from build123d import *

# Parameters (mm, degrees)
BOSS_EXTRUDE1_DEPTH            = 3
SKETCH2_W                      = 2.725
SKETCH2_H                      = 93.5
REVOLVE1_ANGLE                 = 180
SKETCH2_3_W                    = 1.7
SKETCH2_3_H                    = 93.5
M4_CLEARANCE_HOLE1_D           = 4.5
M4_CLEARANCE_HOLE1_CSINK_D     = 4.55
M4_CLEARANCE_HOLE1_CSINK_ANGLE = 90
FILLET1_R                      = 4
FILLET2_R                      = 2.5
CUT_EXTRUDE2_DEPTH             = 5


with BuildPart() as part:
    # Sketch1 → Boss-Extrude1 (new body)
    with BuildSketch(Plane.XY):
        Polygon((-22, 0), (22, 0), (22, -10), (40, -10), (40, -39.5), (24.672961021, -39.5), (12, -71.5), (-12, -71.5), (-24.672961021, -39.5), (-40, -39.5), (-40, -10), (-22, -10), align=None)
    extrude(amount=BOSS_EXTRUDE1_DEPTH)

    # Sketch2 → Revolve1 (revolve)
    with BuildSketch(Plane.XY):
        with Locations((-3.0625, -118.25)):
            Rectangle(SKETCH2_W, SKETCH2_H)
        Polygon((-4.425, -40), (-4.425, -71.5), (-1.7, -71.5), (-1.7, -34), (-4.425, -34), (-4.425, 0), (-10, 0), (-10, -30), align=None)
    revolve(axis=Axis((0, 0, 0), (0, 1, 0)), revolution_arc=REVOLVE1_ANGLE)

    # Sketch2<3> → Cut-Revolve1 (revolve, cut)
    with BuildSketch(Plane.XY):
        with Locations((-0.85, -118.25)):
            Rectangle(SKETCH2_3_W, SKETCH2_3_H)
        Polygon((-1.7, -34), (-1.7, -71.5), (0, -71.5), (0, 0), (-4.425, 0), (-4.425, -34), align=None)
    revolve(axis=Axis((0, 0, 0), (0, -1, 0)), mode=Mode.SUBTRACT)

    # M4 Clearance Hole1 (through all)
    with Locations(Plane.XY.offset(3)):
        with Locations((-35.5, -14.5), (-9, -66.5), (9, -66.5), (35.5, -14.5)):
            CounterSinkHole(M4_CLEARANCE_HOLE1_D / 2, M4_CLEARANCE_HOLE1_CSINK_D / 2, counter_sink_angle=M4_CLEARANCE_HOLE1_CSINK_ANGLE)

    # Fillet1
    # the kernel refuses this fillet: 4 mm, written as the material it adds along each edge
    with BuildSketch(Plane(origin=(0, -34, 0), x_dir=(1, 0, 0), z_dir=(0, 0, -1))) as fillet1_piece_1:
        with BuildLine():
            CenterArc((0.425, -3.791355299), FILLET1_R, 0, 71.412652979)
            Line((1.7, 0), (1.7255, 0.075827106))
            ThreePointArc((1.7255, 0.075827106), (3.0625, 0.08), (4.425, 0.08))
            Line((4.425, 0.08), (4.505, 0))
            Line((4.505, 0), (4.505, -3.791355299))
            Line((4.505, -3.791355299), (4.425, -3.791355299))
        make_face()
    revolve(axis=Axis((0, -34, 0), (0, -1, 0)), revolution_arc=180)

    # Fillet2
    fillet2_edges = [part.edges().sort_by_distance(p)[0] for p in [
        (-22, 0, 1.5),
        (22, 0, 1.5),
        (22, -10, 1.5),
        (40, -10, 1.5),
        (40, -39.5, 1.5),
        (24.672961021, -39.5, 1.5),
        (12, -71.5, 1.5),
        (-12, -71.5, 1.5),
        (-24.672961021, -39.5, 1.5),
        (-40, -39.5, 1.5),
        (-40, -10, 1.5),
        (-22, -10, 1.5),
        (4.121541499, -71.5, 1.610441142),
        (-4.121541499, -71.5, 1.610441142),
    ]]
    fillet(fillet2_edges, radius=FILLET2_R)

    # Sketch9 → Cut-Extrude2 (cut, symmetric)
    with BuildSketch(Plane(origin=(0, 0, 0), x_dir=(0, 0, -1), z_dir=(1, 0, 0))):
        Polygon((-4.425, -162), (4.425, -165), (-4.425, -165), align=None)
    extrude(amount=CUT_EXTRUDE2_DEPTH, both=True, mode=Mode.SUBTRACT)


solid = part.part
Build history of the part. All positions in model axes, mm. A direction names the side the tool comes from. Coordinates: 2 decimals unless noted, no trailing zeros. Order: outer loops, then holes, each group sorted by start corner. A loop starts at its lowest first (then second) coordinate and runs counter-clockwise, first axis right, second up. Notation, with made-up numbers: (-10.75, 9.25) -> (10.25, 9.25) arc R23 cw to (10.25, 28.25) -> close; hole circle Ø11 at (60, 75.5). An arc over 180 degrees is marked (long way). One line per item, written item: value.
(1) Tool access for faces 5 (the cylindrical face through (0.097, -15.316, 4.424)), 6 (the flat face through (-22, -5, 1)), 7 (the flat face through (22, -5, 1)): list every direction of +Z, -Z, +X, -X, +Y, -Y with a clear straight run to the whole face (end or side of a thin tool).
Checked values:
face 5: -Z, +Y
face 6: +Z, -Z, -X, +Y
face 7: +Z, -Z, +X, +Y
(2) Mould opens along Y. For faces 1 (the cylindrical face through (33.42, -15.36, 1.47)), 2 (the flat face through (-9, -71.5, 1)), 3 (the flat face through (40, -25, 1)), 4 (the cylindrical face through (-37.58, -15.36, 1.47)) say: pulls with the +Y half, pulls with the -Y half, needs draft (parallel to the pull), parting line crosses it, or undercut.
Checked values:
face 1: undercut
face 2: pulls with the -Y half
face 3: needs draft
face 4: undercut
(3) Slice it at B-B, the plane x = -29. List the corners of the cut face in (y, z), plus the area to 3 significant figures.
Checked values:
outline: (-39.5, 0) -> (-10, 0) -> (-10, 3) -> (-39.5, 3) -> close
area: 88.5 mm2
(4) Slice it at C-C, the plane y = -147. List the corners of the cut face in (x, z) (3 decimals), plus the area to 3 significant figures.
Checked values:
outline: (-4.425, 0) -> (-1.7, 0) arc R1.7 cw to (1.7, 0) -> (4.425, 0) arc R4.425 ccw to start
area: 26.2 mm2
(5) Slice it at A-A, the plane y = -14.5. List the corners of the cut face in (x, z) (3 decimals), plus the area to 3 significant figures.
Checked values:
outline: (-40, 0) -> (-37.75, 0) -> (-37.75, 2.975) -> (-37.775, 3) -> (-40, 3) -> close; (-33.25, 0) -> (-4.425, 0) arc R4.425 cw to (4.425, 0) -> (33.25, 0) -> (33.25, 2.975) -> (33.225, 3) -> (9.539, 3) arc R10 ccw to (-9.539, 3) -> (-33.225, 3) -> (-33.25, 2.975) -> close; (37.75, 0) -> (40, 0) -> (40, 3) -> (37.775, 3) -> (37.75, 2.975) -> close
area: 280 mm2
(6) Drop flat-ended pins along their axis: pin 1 Ø1.5 at (x, z) = (-31, 2) entering from -Y; pin 2 Ø5 at (y, z) = (-109, 4.5) entering from +X; pin 3 Ø3.5 at (x, z) = (9, 1.5) entering from -Y. Give the stop position or say it passes through.
Checked values:
pin 1: y = -39.5
pin 2: x = 3.95
pin 3: y = -71.5
(7) Probe line 1 (Y direction, x = 35.5, z = 1.15); line 2 (X direction, y = -14.5, z = 1.9); line 3 (Z direction, x = 33, y = -22). List the from-to ranges inside material, lowest first. Write a range as [from, to].
Checked values:
line 1: [-39.5, -16.75], [-12.25, -10]
line 2: [-40, -37.75], [-33.25, -4], [4, 33.25], [37.75, 40]
line 3: [0, 3]
